from build123d import *

# Parameters (mm, degrees)
F0_W      = 64
F0_H      = 46
F1_DEPTH  = 16
F2_W      = 60
F2_H      = 42
F3_DEPTH  = 14
F4_W      = 40
F4_H      = 27
F5_DEPTH  = 25
F6_R      = 2
F7_W      = 2.5
F7_H      = 16
F8_DEPTH  = 20
F9_R      = 1.4317723001
F10_DEPTH = 25
F11_W     = 26
F11_H     = 11
F12_DEPTH = 25
F13_W     = 26
F13_H     = 9
F14_DEPTH = 25
F15_W     = 12
F15_H     = 8
F16_DEPTH = 25
F17_R     = 1


with BuildPart() as f1:
    # F0 (on Top) → F1 (new body)
    with BuildSketch(Plane.XY):
        with Locations((7.1285768165, 0.5159020871)):
            Rectangle(F0_W, F0_H)
    extrude(amount=F1_DEPTH)

    # F2 (on face) → F3 (cut)
    with BuildSketch(Plane.XY.offset(16)):
        with Locations((7.1285768165, 0.5159020871)):
            Rectangle(F2_W, F2_H)
    extrude(amount=-F3_DEPTH, mode=Mode.SUBTRACT)

    # F4 (on face) → F5 (cut)
    with BuildSketch(Plane.XY.offset(2)):
        with Locations((7.1285768165, 3.0159020871)):
            Rectangle(F4_W, F4_H)
    extrude(amount=-F5_DEPTH, mode=Mode.SUBTRACT)

    # F6
    f6_edges = [f1.edges().sort_by_distance(p)[0] for p in [
        (-12.871423, 16.515902, 1),
        (-12.871423, -10.484098, 1),
        (27.128577, -10.484098, 1),
        (27.128577, 16.515902, 1),
    ]]
    fillet(f6_edges, radius=F6_R)

    # F7 (on face) → F8 (join)
    with BuildSketch(Plane.XZ.offset(22.4840979129)):
        with Locations((4.1285768165, 8)):
            Rectangle(F7_W, F7_H)
        with Locations((10.1285768165, 8)):
            Rectangle(F7_W, F7_H)
    extrude(amount=F8_DEPTH)

    # F9 (on face) → F10 (cut)
    with BuildSketch(Plane(origin=(2.8785768165, 0, 0), x_dir=(0, -1, 0), z_dir=(-1, 0, 0))):
        with Locations((34.4840979129, 8)):
            Circle(F9_R)
        with BuildLine():
            ThreePointArc((34.4840979129, 16), (40.1409521624, 13.6568542495), (42.4840979129, 8))
            Line((42.4840979129, 8), (42.4840979129, 16))
            Line((42.4840979129, 16), (34.4840979129, 16))
        make_face()
        with BuildLine():
            Line((42.4840979129, 0), (42.4840979129, 8))
            ThreePointArc((42.4840979129, 8), (40.1409521624, 2.3431457505), (34.4840979129, 0))
            Line((34.4840979129, 0), (42.4840979129, 0))
        make_face()
    extrude(amount=-F10_DEPTH, mode=Mode.SUBTRACT)

    # F11 (on face) → F12 (cut)
    with BuildSketch(Plane.YZ.offset(39.1285768165)):
        with Locations((1.5159020871, 10.5)):
            Rectangle(F11_W, F11_H)
    extrude(amount=-F12_DEPTH, mode=Mode.SUBTRACT)

    # F13 (on face) → F14 (cut)
    with BuildSketch(Plane(origin=(-24.8714231835, 0, 0), x_dir=(0, -1, 0), z_dir=(-1, 0, 0))):
        with Locations((-0.5159020871, 11.5)):
            Rectangle(F13_W, F13_H)
    extrude(amount=-F14_DEPTH, mode=Mode.SUBTRACT)

    # F15 (on face) → F16 (cut)
    with BuildSketch(Plane(origin=(0, 23.5159020871, 0), x_dir=(-1, 0, 0), z_dir=(0, 1, 0))):
        with Locations((10.8714231835, 12)):
            Rectangle(F15_W, F15_H)
    extrude(amount=-F16_DEPTH, mode=Mode.SUBTRACT)

    # F17
    f17_edges = [f1.edges().sort_by_distance(p)[0] for p in [
        (-23.871423, 13.515902, 16),
        (-23.871423, -12.484098, 16),
        (38.128577, 14.515902, 16),
        (38.128577, -11.484098, 16),
        (-23.871423, 13.515902, 7),
        (38.128577, 14.515902, 5),
        (-23.871423, -12.484098, 7),
        (38.128577, -11.484098, 5),
        (-4.871423, 22.515902, 16),
        (-16.871423, 22.515902, 16),
        (-4.871423, 22.515902, 8),
        (-16.871423, 22.515902, 8),
        (2.878577, -22.484098, 8),
        (11.378577, -22.484098, 8),
    ]]
    fillet(f17_edges, radius=F17_R)


solid = f1.part
Here's how the part is built. I have some questions about the finished solid (model axes, mm). A direction names the side the tool comes from. Round coordinates to 2 decimals unless told otherwise and drop trailing zeros. Order: outer loops, then holes, each group sorted by start corner. A loop starts at its lowest first (then second) coordinate and runs counter-clockwise, first axis right, second up. Notation, with made-up numbers: M 11,51.25 L 22,51.25 A6 cw 22,59.25 Z; hole C 17,61.25 d5. An arc over 180 degrees is marked long. Return JSON: item names as keys, results as strings. Group by question number.
1. If we section it at A-A on x = 4.5: List the corners of the cut face in (y, z) for me.
2. I'm going to push flat-ended pins straight in: pin 1 Ø1.1 at (x, z) = (7, 10) entering from -Y; pin 2 Ø1 at (x, y) = (-23.5, 2.5) entering from +Z; pin 3 Ø1.7 at (y, z) = (-34.48, 8) entering from -X; pin 4 Ø2 at (x, y) = (-12.5, 22) entering from +Z. Where does each tip first touch, or does it pass through?
3. If we section it at C-C on x = -14.5: List the corners of the cut face in (y, z) for me, then the cut area to 3 significant figures.
4. On a 3-axis mill with a long thin cutter (end or side, diameter ignored), from which of +Z, -Z, +X, -X, +Y, -Y can I reach the whole of each face in a straight line? I mean faces 1 (the face through (-24, -12.484, 11)), 2 (the face through (-4.871, 23, 12)), 3 (the face through (26.56, 15.91, 0.99)), 4 (the face through (38, 1, 5)). Say none if no direction works.
5. Please list where these lines run through material, in increasing order: probe 1 along X at (y, z) = (-36, 11.75); probe 2 along Y at (x, z) = (17.5, 2.75); probe 3 along X at (y, z) = (-19, 11.25).
6. If we section it at D-D on y = -15: List the corners of the cut face in (x, z) for me, then the cut area to 3 significant figures.
7. If we mould it in two halves opening along X, with no side actions, what happens to faces 5 (the face through (26, -22.484, 8)), 6 (the face through (-11, 23, 8)), 7 (the face through (2.879, -32.9, 7.9)), 8 (the face through (7, -10.484, 1))? For each: pulls with the +X half, pulls with the -X half, needs draft (parallel to the pull), parting line crosses it, or undercut.
8. If we section it at B-B on y = -29: List the corners of the cut face in (x, z) for me.
Reply:
{
 "1": {"outline": "M -34.48,0 L -10.48,0 L -10.48,2 L -20.48,2 L -20.48,16 L -34.48,16 A8 ccw Z; M 16.52,0 L 23.52,0 L 23.52,16 L 21.52,16 L 21.52,2 L 16.52,2 Z; hole C -34.48,8 d2.86"},
 "2": {"pin 1": "y = -22.48", "pin 2": "z = 7", "pin 3": "through", "pin 4": "z = 8"},
 "3": {"outline": "M -22.48,0 L 23.52,0 L 23.52,8 L 21.52,8 L 21.52,2 L -20.48,2 L -20.48,16 L -22.48,16 Z", "area": "132 mm^2"},
 "4": {"face 1": "+Z, -X", "face 2": "+Z, +Y", "face 3": "+Z, -Z", "face 4": "+Z, +X"},
 "5": {"probe 1": "2.88 to 5.38, 8.88 to 11.38", "probe 2": "-22.48 to -20.48, 21.52 to 23.52", "probe 3": "-24.87 to -22.87, 37.13 to 39.13"},
 "6": {"outline": "M -24.87,0 L 39.13,0 L 39.13,16 L 37.13,16 L 37.13,2 L -22.87,2 L -22.87,16 L -24.87,16 Z", "area": "184 mm^2"},
 "7": {"face 5": "needs draft", "face 6": "undercut", "face 7": "pulls with the -X half", "face 8": "undercut"},
 "8": {"outline": "M 2.88,0 L 5.38,0 L 5.38,16 L 2.88,16 Z; M 8.88,0 L 11.38,0 L 11.38,16 L 8.88,16 Z"}
}
